Part model, mm, in its own coordinate system. A direction names the side the tool comes from. Coordinates: 2 decimals unless noted, no trailing zeros. Write each loop counter-clockwise with the first axis right and the second up, starting at its lowest first coordinate (ties: lowest second). Pieces come first, ordered by that corner, then holes. Notation, with made-up numbers: (60, 78.25) -> (76, 78.25) arc R17 cw to (76, 86.25) -> close; hole circle Ø3 at (3, 88). An arc over 180 degrees is marked (long way). Write item = value, one per line.
from build123d import *

# Parameters (mm, degrees)
F1_DEPTH = 7
F2_T     = 2
F3_D     = 8
F4_W     = 5
F4_H     = 2
F5_DEPTH = 2


# Not quite as in the source:
# - a feature of the source that left no trace in its solid (it failed there, or was rolled back) is left out


with BuildPart() as f1:
    # F0 (on Front) → F1 (new body)
    with BuildSketch(Plane.XZ):
        with BuildLine():
            ThreePointArc((0, -13.5), (9.545941546, -9.545941546), (13.5, 0))
            ThreePointArc((13.5, 0), (9.545941546, 9.545941546), (0, 13.5))
            Line((0, 13.5), (0, -13.5))
        make_face()
        with BuildLine():
            ThreePointArc((0, 13.5), (9.545941546, 9.545941546), (13.5, 0))
            ThreePointArc((13.5, 0), (9.545941546, -9.545941546), (0, -13.5))
            Line((0, -13.5), (110, -13.5))
            Line((110, -13.5), (110, 13.5))
            Line((110, 13.5), (0, 13.5))
        make_face()
        with BuildLine():
            Line((0, -13.5), (0, 13.5))
            ThreePointArc((0, 13.5), (-13.5, 0), (0, -13.5))
        make_face()
    extrude(amount=F1_DEPTH)

    # F2
    f2_openings = [f1.faces().sort_by_distance(p)[0] for p in [
        (49.660922, 0, 0),
        (110, -3.5, 0),
    ]]
    offset(amount=F2_T, openings=f2_openings, kind=Kind.INTERSECTION)

    # F3 (through all)
    with Locations(Plane(origin=(0, 0, 0), x_dir=(1, 0, 0), z_dir=(0, 1, 0))):
        with Locations((0, 0)):
            Hole(F3_D / 2)

    # F4 (on face) → F5 (join)
    with BuildSketch(Plane(origin=(0, 0, 0), x_dir=(-1, 0, 0), z_dir=(0, 1, 0))):
        with Locations((-17.5, -14.5)):
            Rectangle(F4_W, F4_H)
        with BuildLine():
            Line((-20, -13.5), (-15, -13.5))
            ThreePointArc((-15, -13.5), (-17.5, -11), (-20, -13.5))
        make_face()
        with Locations((-32.5, -14.5)):
            Rectangle(F4_W, F4_H)
        with BuildLine():
            Line((-35, -13.5), (-30, -13.5))
            ThreePointArc((-30, -13.5), (-32.5, -11), (-35, -13.5))
        make_face()
        with Locations((-47.5, -14.5)):
            Rectangle(F4_W, F4_H)
        with BuildLine():
            Line((-50, -13.5), (-45, -13.5))
            ThreePointArc((-45, -13.5), (-47.5, -11), (-50, -13.5))
        make_face()
        with Locations((-62.5, -14.5)):
            Rectangle(F4_W, F4_H)
        with BuildLine():
            Line((-65, -13.5), (-60, -13.5))
            ThreePointArc((-60, -13.5), (-62.5, -11), (-65, -13.5))
        make_face()
        with Locations((-77.5, -14.5)):
            Rectangle(F4_W, F4_H)
        with BuildLine():
            Line((-80, -13.5), (-75, -13.5))
            ThreePointArc((-75, -13.5), (-77.5, -11), (-80, -13.5))
        make_face()
        with Locations((-17.5, 14.5)):
            Rectangle(F4_W, F4_H)
        with BuildLine():
            ThreePointArc((-20, 13.5), (-17.5, 11), (-15, 13.5))
            Line((-15, 13.5), (-20, 13.5))
        make_face()
        with BuildLine():
            ThreePointArc((-35, 13.5), (-32.5, 11), (-30, 13.5))
            Line((-30, 13.5), (-35, 13.5))
        make_face()
        with Locations((-32.5, 14.5)):
            Rectangle(F4_W, F4_H)
        with BuildLine():
            ThreePointArc((-50, 13.5), (-47.5, 11), (-45, 13.5))
            Line((-45, 13.5), (-50, 13.5))
        make_face()
        with Locations((-47.5, 14.5)):
            Rectangle(F4_W, F4_H)
        with BuildLine():
            ThreePointArc((-65, 13.5), (-62.5, 11), (-60, 13.5))
            Line((-60, 13.5), (-65, 13.5))
        make_face()
        with Locations((-62.5, 14.5)):
            Rectangle(F4_W, F4_H)
        with BuildLine():
            ThreePointArc((-80, 13.5), (-77.5, 11), (-75, 13.5))
            Line((-75, 13.5), (-80, 13.5))
        make_face()
        with Locations((-77.5, 14.5)):
            Rectangle(F4_W, F4_H)
    extrude(amount=F5_DEPTH)


solid = f1.part
Q1. Pin check, flat tips, straight feed: pin 1 (1.6 mm diameter, centred on x = 57, z = -14.5, fed in from +Y); pin 2 (6 mm diameter, centred on y = -2.5, z = -4.5, fed in from -X); pin 3 (1.6 mm diameter, centred on y = 1, z = -14.5, fed in from +X). Stop position of each tip, or through.
Model answer:
pin_1 = 0
pin_2 = -15.43
pin_3 = 80
Q2. Saw through at C-C on y = -2. Give the cut face in (x, z).
Model answer:
outline = (0, -15.5) -> (110, -15.5) -> (110, -13.5) -> (0, -13.5) arc R13.5 cw to (0, 13.5) -> (110, 13.5) -> (110, 15.5) -> (0, 15.5) arc R15.5 ccw to start
Q3. Mould opens along Z. For faces 6 (the face through (33, 2, -13)), 7 (the face through (77.4, 1, -11)), 8 (the face through (77.6, 1, 11)) say: released by +Z, released by -Z, zero draft, split by the parting line, or undercut.
Model answer:
face_6 = zero draft
face_7 = undercut
face_8 = undercut
Q4. Saw through at A-A on z = 0. Give the cut face in (x, y).
Model answer:
outline = (-15.5, -9) -> (-4, -9) -> (-4, -7) -> (-13.5, -7) -> (-13.5, 0) -> (-15.5, 0) -> close; (4, -9) -> (110, -9) -> (110, -7) -> (4, -7) -> close
Q5. Saw through at B-B on x = 100. Give the cut face in (y, z), and give its area (3 significant figures).
Model answer:
outline = (-9, -15.5) -> (0, -15.5) -> (0, -13.5) -> (-7, -13.5) -> (-7, 13.5) -> (0, 13.5) -> (0, 15.5) -> (-9, 15.5) -> close
area = 90.0 mm²
Q6. Probe line 1 (Z direction, x = 17.5, y = -2); line 2 (Z direction, x = 0, y = -7.4); line 3 (X direction, y = 1.5, z = -12.5). List the from-to ranges inside material, lowest first. Write a range as from..to.
Model answer:
line_1 = -15.5..-13.5, 13.5..15.5
line_2 = -15.5..-4, 4..15.5
line_3 = 15.21..19.79, 30.21..34.79, 45.21..49.79, 60.21..64.79, 75.21..79.79
Q7. Saw through at D-D on x = 32.5. Give the cut face in (y, z), and give its area (3 significant figures).
Model answer:
outline = (-9, -15.5) -> (2, -15.5) -> (2, -11) -> (0, -11) -> (0, -13.5) -> (-7, -13.5) -> (-7, 13.5) -> (0, 13.5) -> (0, 11) -> (2, 11) -> (2, 15.5) -> (-9, 15.5) -> close
area = 108 mm²
Q8. Which spindle directions (+Z, -Z, +X, -X, +Y, -Y) get a long thin tool onto all of the face, cutting with end or side? Do faces 1 (the face through (25, 0, -14)), 2 (the face through (18, 2, 13)), 3 (the face through (15, 1, 14)), 4 (the face through (54, -3, -13.5)), 5 (the face through (47.4, 1, -11)). Say none if no direction does.
Model answer:
face_1 = +Z, -Z, +Y
face_2 = +Z, -Z, +X, -X, +Y
face_3 = +Z, -Z, -X, +Y
face_4 = +X
face_5 = +Y
